Input: part model. Units: mm. Frame: model coordinates. Coordinates: 2 decimals unless noted, no trailing zeros. Order: outer loops, then holes, each group sorted by start corner. A loop starts at its lowest first (then second) coordinate and runs counter-clockwise, first axis right, second up. Notation, with made-up numbers: M 55.5,29.5 L 108.5,29.5 A22 ccw 108.5,35.5 Z; hole C 47,-35.75 d3. An arc over 180 degrees is marked long. Answer in a Markdown table with one row per item.
from build123d import *

# Parameters (mm, degrees)
SKETCH_1_W      = 55.3
SKETCH_1_H      = 46.5
SKETCH_1_R      = 1.6
EXTRUDE_1_DEPTH = 2
FILLET_1_R      = 2


with BuildPart() as part:
    # 草图1 → 凸台-拉伸1 (new body)
    with BuildSketch(Plane(origin=(0, 0, 0), x_dir=(1, 0, 0), z_dir=(0, 1, 0))):
        Rectangle(SKETCH_1_W, SKETCH_1_H)
        with Locations(Location((11.65, 13.25, 0), (0, 0, 270))):
            Circle(SKETCH_1_R, mode=Mode.SUBTRACT)
        with Locations(Location((-8.35, 13.25, 0), (0, 0, 270))):
            Circle(SKETCH_1_R, mode=Mode.SUBTRACT)
        with Locations(Location((24.65, 20.25, 0), (0, 0, 270))):
            Circle(SKETCH_1_R, mode=Mode.SUBTRACT)
        with Locations(Location((-24.65, 20.25, 0), (0, 0, 270))):
            Circle(SKETCH_1_R, mode=Mode.SUBTRACT)
        with Locations(Location((-24.65, -19.95, 0), (0, 0, 270))):
            Circle(SKETCH_1_R, mode=Mode.SUBTRACT)
        with Locations(Location((24.65, -19.95, 0), (0, 0, 270))):
            Circle(SKETCH_1_R, mode=Mode.SUBTRACT)
        Polygon((-3.107609479, 0), (-22.65, 16.432570691), (-22.65, -16.432570691), align=None, mode=Mode.SUBTRACT)
        Polygon((0, -2.613089345), (-18.596153962, -18.25), (18.596153962, -18.25), align=None, mode=Mode.SUBTRACT)
        Polygon((3.107609479, 0), (22.65, 16.432570691), (22.65, -16.432570691), align=None, mode=Mode.SUBTRACT)
    extrude(amount=EXTRUDE_1_DEPTH)

    # 圆角1
    fillet_1_edges = [part.edges().sort_by_distance(p)[0] for p in [
        (-22.65, 1, 16.432570691),
        (-3.107609479, 1, 0),
        (-22.65, 1, -16.432570691),
        (18.596153962, 1, 18.25),
        (0, 1, 2.613089345),
        (-18.596153962, 1, 18.25),
        (3.107609479, 1, 0),
        (22.65, 1, 16.432570691),
        (22.65, 1, -16.432570691),
        (27.65, 1, 23.25),
        (-27.65, 1, 23.25),
        (-27.65, 1, -23.25),
        (27.65, 1, -23.25),
    ]]
    fillet(fillet_1_edges, radius=FILLET_1_R)


solid = part.part
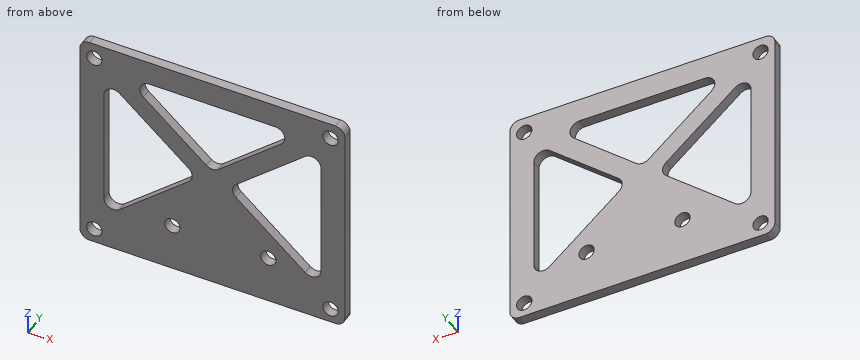
1) Contact query for a flat-ended pin moving along its axis: pin 1 (3 mm diameter, centred on x = -24.65, z = 19.95, fed in from +Y). Output: stop coordinate, or through.
Resolved:
| item | result |
|---|---|
| pin 1 | passes through |
2) Cut plane C-C, the plane z = -20.25. Output: boundary loops of the cut face in (x, y).
Resolved:
| item | result |
|---|---|
| outline | M -27.65,0 L -26.25,0 L -26.25,2 L -27.65,2 Z; M -23.05,0 L 23.05,0 L 23.05,2 L -23.05,2 Z; M 26.25,0 L 27.65,0 L 27.65,2 L 26.25,2 Z |
3) Material intervals for probe 1 along X at (y, z) = (1.3, -20.25); probe 2 along X at (y, z) = (0.35, 14.5); probe 3 along Z at (x, y) = (-14.5, 0.85), sorted ascending.
Resolved:
| item | result |
|---|---|
| probe 1 | x = -27.65 to -26.25, -23.05 to 23.05, 26.25 to 27.65 |
| probe 2 | x = -27.65 to -14.14, 14.14 to 27.65 |
| probe 3 | z = -23.25 to -9.58, 9.58 to 14.81, 17.69 to 23.25 |
4) Cut plane A-A, the plane y = 0.3. State how many separate pieces and enclosed holes the cut face has, and give its area (3 significant figures).
Resolved:
| item | result |
|---|---|
| separate pieces | 1 |
| enclosed holes | 9 |
| area | 1,620 mm2 |
5) Cut plane B-B, the plane x = -24.65. Output: boundary loops of the cut face in (y, z), and give its area (3 significant figures).
Resolved:
| item | result |
|---|---|
| outline | M 0,-23.25 L 2,-23.25 L 2,-21.85 L 0,-21.85 Z; M 0,-18.65 L 2,-18.65 L 2,18.35 L 0,18.35 Z; M 0,21.55 L 2,21.55 L 2,23.25 L 0,23.25 Z |
| area | 80.2 mm2 |
6) Cut plane D-D, the plane x = -2. Output: boundary loops of the cut face in (y, z), and give its area (3 significant figures).
Resolved:
| item | result |
|---|---|
| outline | M 0,-23.25 L 2,-23.25 L 2,4.29 L 0,4.29 Z; M 0,18.25 L 2,18.25 L 2,23.25 L 0,23.25 Z |
| area | 65.1 mm2 |
